Part print with two shaded views. Sizes in mm from the minimum x, y, z corner. A direction names the side the tool comes from. Coordinates: 2 decimals unless noted, no trailing zeros. Loops run counter-clockwise (first coordinate to the right, second up) from the corner with the lowest first, then second, coordinate; pieces in that order, holes last.
Item 1: Cut at B-B (z = 42.5). List the corners of the cut face in (x, y).
Item 2: Cut at C-C (y = 68.5). List the corners of the cut face in (x, z), and give its area (3 significant figures).
Item 3: Flat gauge pins, fed straight in: pin 1 (2 mm diameter, centred on x = 26.5, z = 24.5, fed in from -Y); pin 2 (1.5 mm diameter, centred on x = 26, y = 70, fed in from -Z); pin 3 (5 mm diameter, centred on x = 40, y = 62.5, fed in from -Z); pin 4 (16 mm diameter, centred on x = 42.5, z = 75, fed in from +Y). Where does each tip first touch, or does it go through?
Item 4: 3-axis set-ups, long thin cutter, end or side, ignore diameter. For the marked faces 4 and 5: which of +Z, -Z, +X, -X, +Y, -Y reach the whole face in a straight line?
Item 5: Drill centre lines: line 1 along X through (y, z) = (74, 42); line 2 along Y through (x, z) = (25.5, 28); line 3 along X through (y, z) = (78, 10). Where is each one in solid material? Low to high.
Item 6: Cut at D-D (x = 71.5). List the corners of the cut face in (y, z).
Item 7: Cut at A-A (x = 42.5). List the corners of the cut face in (y, z).
Item 8: Mould opens along Z. For the marked faces 1, 2 and 3 say: released by +Z, released by -Z, zero draft, split by the parting line, or undercut.
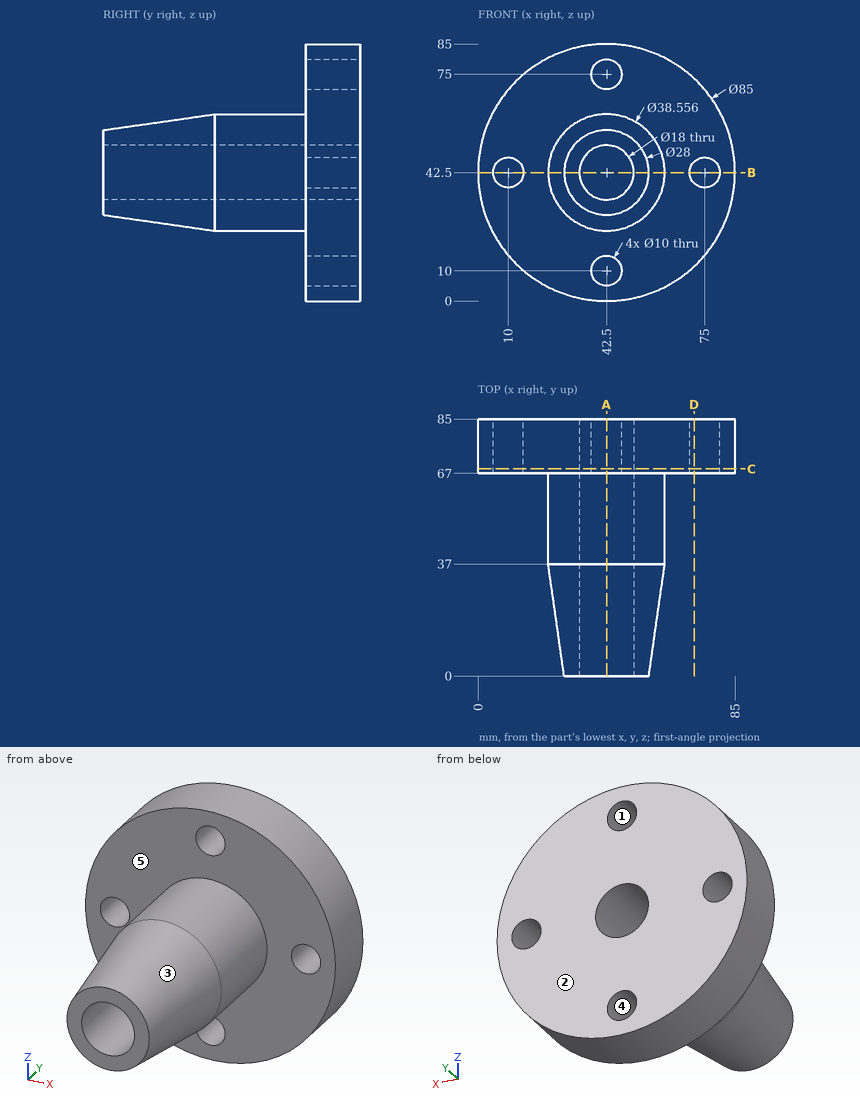
Filled sheet:
1. outline: (0, 67) - (5, 67) - (5, 85) - (0, 85) - close; (15, 67) - (23.22, 67) - (23.22, 37) - (28.5, 0) - (33.5, 0) - (33.5, 85) - (15, 85) - close; (51.5, 0) - (56.5, 0) - (61.78, 37) - (61.78, 67) - (70, 67) - (70, 85) - (51.5, 85) - close; (80, 67) - (85, 67) - (85, 85) - (80, 85) - close
2. outline: circle Ø85 at (42.5, 42.5); hole circle Ø10 at (10, 42.5); hole circle Ø18 at (42.5, 42.5); hole circle Ø10 at (42.5, 10); hole circle Ø10 at (42.5, 75); hole circle Ø10 at (75, 42.5)
2. area: 5,110 mm2
3. pin 1: stops at y = 67
3. pin 2: stops at z = 3.03
3. pin 3: stops at z = 23.22
3. pin 4: stops at y = 85
4. face 4: +Y, -Y
4. face 5: -Y
5. line 1: x = 0 to 5.03, 14.97 to 33.51, 51.49 to 70.03, 79.97 to 85
5. line 2: y = 67 to 85
5. line 3: x = 15.11 to 37.5, 47.5 to 69.89
6. outline: (67, 11.43) - (85, 11.43) - (85, 38.93) - (67, 38.93) - close; (67, 46.07) - (85, 46.07) - (85, 73.57) - (67, 73.57) - close
7. outline: (0, 28.5) - (37, 23.22) - (67, 23.22) - (67, 15) - (85, 15) - (85, 33.5) - (0, 33.5) - close; (0, 51.5) - (85, 51.5) - (85, 70) - (67, 70) - (67, 61.78) - (37, 61.78) - (0, 56.5) - close; (67, 0) - (85, 0) - (85, 5) - (67, 5) - close; (67, 80) - (85, 80) - (85, 85) - (67, 85) - close
8. face 1: undercut
8. face 2: zero draft
8. face 3: split by the parting line
